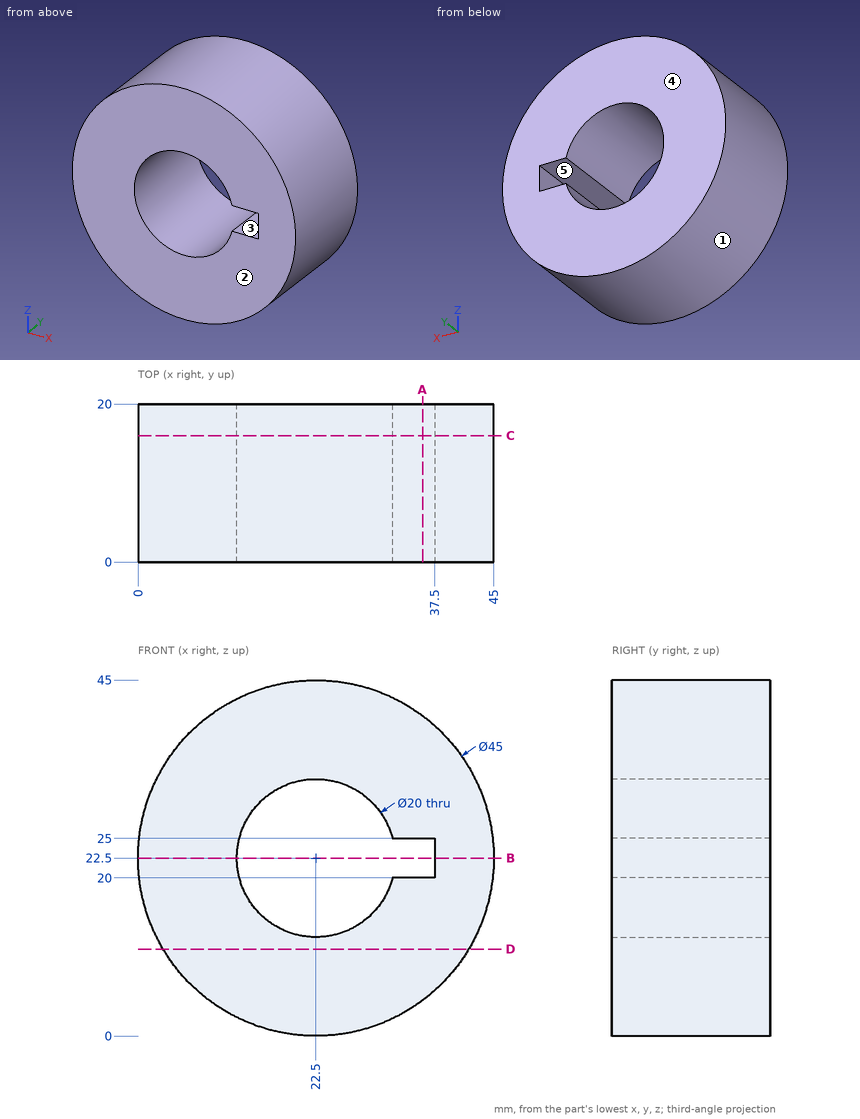
For this review, use the dimensioned drawing (mm, ordinates from the lowest corner) and the shaded views. A direction names the side the tool comes from. Give positions to 0.01 mm unless a question says otherwise; leave off trailing zeros. Order: outer loops, then holes, each group sorted by start corner. A loop starts at its lowest first (then second) coordinate and runs counter-clockwise, first axis right, second up.
1. Add section B-B, the plane z = 22.5. State the section outline as (x, y) points.
Solution:
outline: (0, 0) - (12.5, 0) - (12.5, 20) - (0, 20) - close; (37.5, 0) - (45, 0) - (45, 20) - (37.5, 20) - close
2. For pin 1 Ø6 at (x, y) = (33.5, 6) entering from +Z; pin 2 Ø4 at (x, y) = (40.5, 13) entering from -Z; pin 3 Ø2 at (y, z) = (17.5, 39.5) entering from -X; pin 4 Ø10 at (x, z) = (20, 19.5) entering from +Y, all flat-tipped, find the tip position at first contact; note any pin that passes through.
Solution:
pin 1: stops at z = 43.53
pin 2: stops at z = 6.68
pin 3: stops at x = 6.68
pin 4: passes through
3. To check wall thickness, follow L1, parallel to Z at x = 22.5, y = 15.25; L2, parallel to X at y = 12, z = 22.5; L3, parallel to Z at x = 20, y = 12.25. State the ranges of each line that lie inside material, in increasing order.
Solution:
L1: z = 0 to 12.5, 32.5 to 45
L2: x = 0 to 12.5, 37.5 to 45
L3: z = 0.14 to 12.82, 32.18 to 44.86
4. Add section D-D, the plane z = 11. State the section outline as (x, y) points.
Solution:
outline: (3.16, 0) - (41.84, 0) - (41.84, 20) - (3.16, 20) - close
5. Add section A-A, the plane x = 36. State the section outline as (y, z) points.
Solution:
outline: (0, 4.5) - (20, 4.5) - (20, 20) - (0, 20) - close; (0, 25) - (20, 25) - (20, 40.5) - (0, 40.5) - close
6. Add section C-C, the plane y = 16. State the section outline as (x, z) points, then the cut area to 3 significant figures.
Solution:
outline: circle Ø45 at (22.5, 22.5); hole (32.18, 20) - (37.5, 20) - (37.5, 25) - (32.18, 25) arc R10 ccw (long way) to start
area: 1,250 mm2
7. Tool access review of the marked faces 4 and 5: name each direction out of +Z, -Z, +X, -X, +Y, -Y from which nothing blocks a thin tool from reaching the whole face with its end or side.
Solution:
face 4: +Z, -Z, +X, -X, +Y
face 5: +Y, -Y
8. Mouldability with a two-part tool opening along X and no side actions: class the marked faces 1, 2 and 3 as +X half, -X half, draft (parallel to the pull), parting line (faces both ways), or undercut.
Solution:
face 1: parting line
face 2: draft
face 3: undercut
